```python
from build123d import *

# Parameters (mm, degrees)
F0_W      = 22.8
F0_H      = 12.31
F1_DEPTH  = 22.26
F2_R      = 6.155
F3_DEPTH  = 4.25
F4_R      = 2.625
F5_DEPTH  = 4.25
F6_W      = 2.5
F6_H      = 12.31
F7_DEPTH  = 5
F8_W      = 2.25
F8_H      = 12.31
F9_DEPTH  = 5
F10_R     = 2.5
F11_DEPTH = 2.68
F12_R     = 1
F13_DEPTH = 25


with BuildPart() as f1:
    # F0 (on Front) → F1 (new body)
    with BuildSketch(Plane.XZ):
        Rectangle(F0_W, F0_H)
    extrude(amount=F1_DEPTH)

    # F2 (on face) → F3 (join)
    with BuildSketch(Plane.XZ.offset(22.26)):
        with Locations((-5.245, 0)):
            Circle(F2_R)
    extrude(amount=F3_DEPTH)

    # F4 (on face) → F5 (join)
    with BuildSketch(Plane.XZ.offset(22.26)):
        Circle(F4_R)
    extrude(amount=F5_DEPTH)

    # F6 (on face) → F7 (join)
    with BuildSketch(Plane(origin=(-11.4, 0, 0), x_dir=(0, -1, 0), z_dir=(-1, 0, 0))):
        with Locations((16.69, 0)):
            Rectangle(F6_W, F6_H)
    extrude(amount=F7_DEPTH)

    # F8 (on face) → F9 (join)
    with BuildSketch(Plane.YZ.offset(11.4)):
        with Locations((-16.815, 0)):
            Rectangle(F8_W, F8_H)
    extrude(amount=F9_DEPTH)

    # F10 (on face) → F11 (join)
    with BuildSketch(Plane.XZ.offset(26.51)):
        with Locations((-5.245, 0)):
            Circle(F10_R)
    extrude(amount=F11_DEPTH)

    # F12 (on face) → F13 (cut)
    with BuildSketch(Plane.XZ.offset(17.94)):
        with Locations((-14, 0)):
            Circle(F12_R)
        with Locations((14, 0)):
            Circle(F12_R)
    extrude(amount=-F13_DEPTH, mode=Mode.SUBTRACT)


solid = f1.part
```
Can you work these out from the model? Positions are in its coordinate system, mm. A direction names the side the tool comes from. Round coordinates to 2 decimals unless told otherwise and drop trailing zeros. Loops run counter-clockwise (first coordinate to the right, second up) from the corner with the lowest first, then second, coordinate; pieces in that order, holes last. Notation, with made-up numbers: M 11.5,26.5 L 66.5,26.5 A9 cw 66.5,31.5 Z; hole C -34,32 d4. An arc over 180 degrees is marked long. Answer in a Markdown table with one row per item.
1. Please list where these lines run through material, in increasing order: line 1 (Z direction, x = 14, y = -16.75) (3 decimals); line 2 (Y direction, x = 7, z = 1); line 3 (Y direction, x = -1.5, z = 0.75). Write a range as from..to.
Established:
| item | result |
|---|---|
| line 1 | -6.155..-1, 1..6.155 |
| line 2 | -22.26..0 |
| line 3 | -26.51..0 |
2. If we section it at C-C, the plane x = 14: Please give me the cut outline in (y, z) (3 decimals).
Established:
| item | result |
|---|---|
| outline | M -17.94,-6.155 L -15.69,-6.155 L -15.69,-1 L -17.94,-1 Z; M -17.94,1 L -15.69,1 L -15.69,6.155 L -17.94,6.155 Z |
3. Thinking about a two-plate mould opening in X: for faces 4 (the face through (-13, -17, 0)), 5 (the face through (15, -17, 0)), 6 (the face through (-10, -22.26, 5)), 7 (the face through (11.4, -8, 0)), which applies, pulls with the +X half, pulls with the -X half, needs draft (parallel to the pull), parting line crosses it, or undercut?
Established:
| item | result |
|---|---|
| face 4 | undercut |
| face 5 | undercut |
| face 6 | needs draft |
| face 7 | pulls with the +X half |
4. If we section it at B-B, the plane z = 2: Please give me the cut outline in (x, y) (3 decimals), plus the area to 3 significant figures.
Established:
| item | result |
|---|---|
| outline | M -16.4,-17.94 L -11.4,-17.94 L -11.4,-22.26 L -11.066,-22.26 L -11.066,-26.51 L -6.745,-26.51 L -6.745,-29.19 L -3.745,-29.19 L -3.745,-26.51 L 1.7,-26.51 L 1.7,-22.26 L 11.4,-22.26 L 11.4,-17.94 L 16.4,-17.94 L 16.4,-15.69 L 11.4,-15.69 L 11.4,0 L -11.4,0 L -11.4,-15.44 L -16.4,-15.44 Z |
| area | 594 mm² |
5. On a 3-axis mill with a long thin cutter (end or side, diameter ignored), from which of +Z, -Z, +X, -X, +Y, -Y can I reach the whole of each face in a straight line? I mean faces 1 (the face through (-10, -22.26, -5)), 2 (the face through (-12.8, -17.94, -0.1)), 3 (the face through (-2.9, -26.51, -1.3)). Say none if no direction works.
Established:
| item | result |
|---|---|
| face 1 | -Z, -X, -Y |
| face 2 | +Z, -Z, -X, -Y |
| face 3 | -Y |
6. If we section it at A-A, the plane x = -14: Please give me the cut outline in (y, z) (3 decimals), plus the area to 3 significant figures.
Established:
| item | result |
|---|---|
| outline | M -17.94,-6.155 L -15.44,-6.155 L -15.44,-1 L -17.94,-1 Z; M -17.94,1 L -15.44,1 L -15.44,6.155 L -17.94,6.155 Z |
| area | 25.8 mm² |
7. If we section it at D-D, the plane y = -21.5: Please give me the cut outline in (x, z) (3 decimals), plus the area to 3 significant figures.
Established:
| item | result |
|---|---|
| outline | M -11.4,-6.155 L 11.4,-6.155 L 11.4,6.155 L -11.4,6.155 Z |
| area | 281 mm² |
8. I'm going to push flat-ended pins straight in: pin 1 Ø2 at (y, z) = (-11.5, 5) entering from +X; pin 2 Ø3.5 at (x, z) = (2, 2) entering from -Y; pin 3 Ø2 at (y, z) = (-20.5, -2) entering from -X; pin 4 Ø1.2 at (x, z) = (-14, 0) entering from -Y. Where does each tip first touch, or does it pass through?
Established:
| item | result |
|---|---|
| pin 1 | x = 11.4 |
| pin 2 | y = -26.51 |
| pin 3 | x = -11.4 |
| pin 4 | through |
